```python
from build123d import *

# Parameters (mm, degrees)
F0_R     = 8.0840946313
F0_R_2   = 9.0306543007
F1_DEPTH = 25.4
F2_W     = 36.0785173252
F2_H     = 36.8336421636
F3_DEPTH = 25.4
F5_DEPTH = 36.8346421636
F6_R     = 7.6188514612
F7_DEPTH = 72.3091809102


with BuildPart() as f1:
    # F0 (on Top) → F1 (new body)
    with BuildSketch(Plane.XY):
        with BuildLine():
            Line((33.0527582523, 18.4168210818), (-39.409391582, 18.4168210818))
            ThreePointArc((-39.409391582, 18.4168210818), (-57.8262126638, 0), (-39.409391582, -18.4168210818))
            Line((-39.409391582, -18.4168210818), (33.0527582523, -18.4168210818))
            ThreePointArc((33.0527582523, -18.4168210818), (51.4695793341, 0), (33.0527582523, 18.4168210818))
        make_face()
        with Locations((-39.409391582, 0)):
            Circle(F0_R, mode=Mode.SUBTRACT)
        with Locations((33.0527582523, 0)):
            Circle(F0_R_2, mode=Mode.SUBTRACT)
    extrude(amount=F1_DEPTH)

    # F2 (on face) → F3 (join)
    with BuildSketch(Plane.XY.offset(25.4)):
        with Locations((-3.5572904162, 0)):
            Rectangle(F2_W, F2_H)
    extrude(amount=F3_DEPTH)

    # F4 (on face) → F5 (cut, through all)
    with BuildSketch(Plane.XZ.offset(18.4168210818)):
        with BuildLine():
            Line((-7.9562223055, 50.8), (-7.9562223055, 12.6487202942))
            ThreePointArc((-7.9562223055, 12.6487202942), (0, 4.6924979887), (7.9562223055, 12.6487202942))
            Line((7.9562223055, 12.6487202942), (7.9562223055, 50.8))
            Line((7.9562223055, 50.8), (-7.9562223055, 50.8))
        make_face()
    extrude(amount=-F5_DEPTH, mode=Mode.SUBTRACT)

    # F6 (on face) → F7 (cut, through all)
    with BuildSketch(Plane.YZ.offset(14.4819682464)):
        with Locations((0, 38.9469414949)):
            Circle(F6_R)
    extrude(amount=-F7_DEPTH, mode=Mode.SUBTRACT)


solid = f1.part
```
Geometry check sheet. Reference: the model listing, model coordinates, mm. A direction names the side the tool comes from. Coordinates: 2 decimals unless noted, no trailing zeros. Write each loop counter-clockwise with the first axis right and the second up, starting at its lowest first coordinate (ties: lowest second). Pieces come first, ordered by that corner, then holes. Notation, with made-up numbers: M 85,69 L 120,69 A21 ccw 120,106 Z; hole C -12,-11 d4. An arc over 180 degrees is marked long. One line per item, written item: value. Start each with the question number.
(1) Sectioned sample at D-D, the plane z = 32.5. Enter the section's corners in (x, y).
(2) Tool access check on faces 1 (the face through (14.482, -4, 32)), 2 (the face through (-32, -4, 25.4)), 3 (the face through (7.956, 0, 27)). Record the directions out of +Z, -Z, +X, -X, +Y, -Y that give a thin tool (end or side, any length) a straight path to the whole face; none if there is none.
(3) Sectioned sample at B-B, the plane z = 8.5. Enter the section's corners in (x, y).
(4) Release check for a two-part mould opening along Z. For faces 4 (the face through (11.26, -1.65, 31.51)), 5 (the face through (-14.68, -1.65, 31.51)), 6 (the face through (-7.956, 0, 28)), 7 (the face through (-0.175, -0.258, 4.694)) record: released by +Z, released by -Z, zero draft, split by the parting line, or undercut.
(5) Sectioned sample at A-A, the plane y = 0. Enter the section's corners in (x, z).
(6) Depth check by flat-ended pin: pin 1 (10 mm diameter, centred on y = 9, z = 7.5, fed in from +X); pin 2 (11 mm diameter, centred on y = -3.5, z = 34, fed in from +X); pin 3 (20.5 mm diameter, centred on y = -8.5, z = 34, fed in from +X). Enter the tip coordinate at first touch or a pass-through.
(7) Sectioned sample at C-C, the plane x = -45. Enter the section's corners in (y, z), and give its area (3 significant figures).
(8) Scan lines: line 1 along X through (y, z) = (9, 31.5); line 2 along X through (y, z) = (2.5, 21.5); line 3 along Z through (x, y) = (-13, 0). Record each from-to range of solid material in increasing order. Write a range as [from, to].
Filled sheet:
1. outline: M -21.6,-18.42 L -7.96,-18.42 L -7.96,-4.06 L -21.6,-4.06 Z; M -21.6,4.06 L -7.96,4.06 L -7.96,18.42 L -21.6,18.42 Z; M 7.96,-18.42 L 14.48,-18.42 L 14.48,-4.06 L 7.96,-4.06 Z; M 7.96,4.06 L 14.48,4.06 L 14.48,18.42 L 7.96,18.42 Z
2. face 1: +Z, +X, +Y, -Y
2. face 2: +Z, -X, +Y, -Y
2. face 3: +Z, +Y, -Y
3. outline: M -39.41,-18.42 L -6.79,-18.42 L -6.79,18.42 L -39.41,18.42 A18.42 ccw Z; M 6.79,-18.42 L 33.05,-18.42 A18.42 ccw 33.05,18.42 L 6.79,18.42 Z; hole C -39.41,0 d16.17; hole C 33.05,0 d18.06
4. face 4: undercut
4. face 5: undercut
4. face 6: zero draft
4. face 7: released by +Z
5. outline: M -57.83,0 L -47.49,0 L -47.49,25.4 L -57.83,25.4 Z; M -31.33,0 L 24.02,0 L 24.02,25.4 L 14.48,25.4 L 14.48,31.33 L 7.96,31.33 L 7.96,12.65 A7.96 cw -7.96,12.65 L -7.96,31.33 L -21.6,31.33 L -21.6,25.4 L -31.33,25.4 Z; M -21.6,46.57 L -7.96,46.57 L -7.96,50.8 L -21.6,50.8 Z; M 7.96,46.57 L 14.48,46.57 L 14.48,50.8 L 7.96,50.8 Z; M 42.08,0 L 51.47,0 L 51.47,25.4 L 42.08,25.4 Z
6. pin 1: x = 51.03
6. pin 2: x = 14.48
6. pin 3: x = 51.24
7. outline: M -17.55,0 L -5.84,0 L -5.84,25.4 L -17.55,25.4 Z; M 5.84,0 L 17.55,0 L 17.55,25.4 L 5.84,25.4 Z
7. area: 595 mm²
8. line 1: [-21.6, -7.96], [7.96, 14.48]
8. line 2: [-57.66, -47.1], [-31.72, -7.96], [7.96, 24.38], [41.73, 51.3]
8. line 3: [0, 31.33], [46.57, 50.8]
